Can you work these out from the model? Positions are in its coordinate system, mm. Round coordinates to 2 decimals unless told otherwise and drop trailing zeros. Write each loop counter-clockwise with the first axis right and the second up, starting at its lowest first coordinate (ties: lowest second). Pieces come first, ordered by that corner, then holes. Notation, with made-up numbers: (64.5, 27.25) - (91.5, 27.25) arc R14 cw to (91.5, 52.25) - close; hole circle Ø9 at (27, -8.5). An arc over 180 degrees is marked (long way). One line per item, written item: value. Start each with the question number.
(1) If I drill on L1, parallel to X at y = -85.5, z = 2.25; L2, parallel to Y at x = 85, z = 16.25; L3, parallel to Y at x = -191.5, z = 15.5, over which ranges is the centre line in solid material (lowest first)? Write a range as from..to.
(2) I'm going to push flat-ended pins straight in: pin 1 Ø10 at (y, z) = (51, 7) entering from -X; pin 2 Ø10 at (x, z) = (-198, 13) entering from -Y. Where does each tip first touch, or does it pass through?
(3) I want a section at C-C on z = 3.5. List the corners of the cut face in (x, y) for me, plus the area to 3 significant figures.
(4) I want a section at A-A on y = -12.5. List the corners of the cut face in (x, z) for me, plus the area to 3 significant figures.
(5) I want a section at B-B on x = 117. List the corners of the cut face in (y, z) for me.
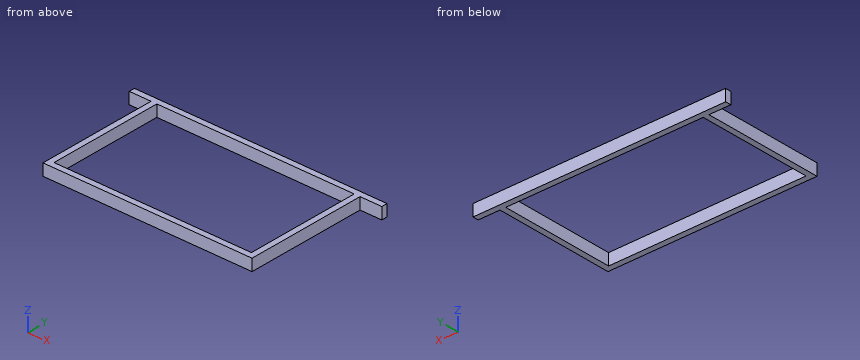
from build123d import *

# Parameters (mm, degrees)
SKETCH1_W           = 360
SKETCH1_H           = 218
SKETCH1_W_2         = 340
SKETCH1_H_2         = 198
SKETCH1_W_3         = 37.5
SKETCH1_H_3         = 10
BOSS_EXTRUDE1_DEPTH = 20


with BuildPart() as part:
    # Sketch1 → Boss-Extrude1 (new body)
    with BuildSketch(Plane.XY):
        Rectangle(SKETCH1_W, SKETCH1_H)
        Rectangle(SKETCH1_W_2, SKETCH1_H_2, mode=Mode.SUBTRACT)
        with Locations((-198.75, 104)):
            Rectangle(SKETCH1_W_3, SKETCH1_H_3)
        with Locations((198.75, 104)):
            Rectangle(SKETCH1_W_3, SKETCH1_H_3)
    extrude(amount=BOSS_EXTRUDE1_DEPTH)


solid = part.part
Established:
1. L1: -180..-170, 170..180
1. L2: -109..-99, 99..109
1. L3: 99..109
2. pin 1: x = -180
2. pin 2: y = 99
3. outline: (-217.5, 99) - (-180, 99) - (-180, -109) - (180, -109) - (180, 99) - (217.5, 99) - (217.5, 109) - (-217.5, 109) - close; hole (-170, -99) - (170, -99) - (170, 99) - (-170, 99) - close
3. area: 11,900 mm2
4. outline: (-180, 0) - (-170, 0) - (-170, 20) - (-180, 20) - close; (170, 0) - (180, 0) - (180, 20) - (170, 20) - close
4. area: 400 mm2
5. outline: (-109, 0) - (-99, 0) - (-99, 20) - (-109, 20) - close; (99, 0) - (109, 0) - (109, 20) - (99, 20) - close
